```python
from build123d import *

# Parameters (mm, degrees)
ESBO_O1_W                = 30
ESBO_O1_H                = 22.5248
RESSALTO_EXTRUS_O1_DEPTH = 12.7
ESBO_O2_W                = 9.2624
ESBO_O2_H                = 20
CORTE_EXTRUS_O1_DEPTH    = 13.7
ESBO_O3_W                = 9.2624
ESBO_O3_H                = 20
CORTE_EXTRUS_O2_DEPTH    = 13.7
FURO1_D                  = 4.9784
FURO1_DEPTH              = 10
FURO1_CBORE_D            = 7.9375
FURO1_CBORE_DEPTH        = 4.1656
ESBO_O8_R                = 1.25
CORTE_EXTRUS_O3_DEPTH    = 10


with BuildPart() as part:
    # Esboço1 → Ressalto-extrusão1 (new body)
    with BuildSketch(Plane(origin=(0, 0, 0), x_dir=(0, -1, 0), z_dir=(-1, 0, 0))):
        with Locations((15, 11.2624)):
            Rectangle(ESBO_O1_W, ESBO_O1_H)
    extrude(amount=-RESSALTO_EXTRUS_O1_DEPTH)

    # Esboço2 → Corte-extrusão1 (cut, through all)
    with BuildSketch(Plane(origin=(12.7, 0, 0), x_dir=(0, 0, -1), z_dir=(1, 0, 0))):
        with Locations((-4.6312, -20)):
            Rectangle(ESBO_O2_W, ESBO_O2_H)
    extrude(amount=-CORTE_EXTRUS_O1_DEPTH, mode=Mode.SUBTRACT)

    # Esboço3 → Corte-extrusão2 (cut, through all)
    with BuildSketch(Plane(origin=(12.7, 0, 0), x_dir=(0, 0, -1), z_dir=(1, 0, 0))):
        with Locations((-17.8936, -20)):
            Rectangle(ESBO_O3_W, ESBO_O3_H)
    extrude(amount=-CORTE_EXTRUS_O2_DEPTH, mode=Mode.SUBTRACT)

    # Furo1
    with Locations(Plane(origin=(0, -10, 0), x_dir=(-1, 0, 0), z_dir=(0, -1, 0))):
        with Locations((-6.35, -4.6312), (-6.35, -17.8936)):
            CounterBoreHole(FURO1_D / 2, FURO1_CBORE_D / 2, FURO1_CBORE_DEPTH, depth=FURO1_DEPTH)

    # Esboço8 → Corte-extrusão3 (cut)
    with BuildSketch(Plane.XY.offset(13.2624)):
        with Locations((6.35, -15.143672471)):
            Circle(ESBO_O8_R)
        with Locations((6.35, -23.520600125)):
            Circle(ESBO_O8_R)
    extrude(amount=-CORTE_EXTRUS_O3_DEPTH, mode=Mode.SUBTRACT)


solid = part.part
```
Can you work these out from the model? Positions are in its coordinate system, mm. A direction names the side the tool comes from. Coordinates: 2 decimals unless noted, no trailing zeros. Loops run counter-clockwise (first coordinate to the right, second up) from the corner with the lowest first, then second, coordinate; pieces in that order, holes last. Notation, with made-up numbers: M -5.5,20.5 L 8.5,20.5 A29 cw 8.5,42.5 Z; hole C 59.25,4 d1. An arc over 180 degrees is marked long. Put each result on its own line as item: value. Start each with the question number.
(1) Will these pins go through, and if not, where does the flat tip stop? pin 1 Ø2.5 at (x, z) = (4.5, 18) entering from -Y; pin 2 Ø2 at (x, y) = (5, -15) entering from +Z; pin 3 Ø3 at (x, z) = (9, 19) entering from -Y.
(2) We'd pull the mould along Z, two halves only. Please class faces 4 (the face through (6, -5, 22.525)), 5 (the face through (12.7, -8, 11)), 6 (the face through (3.8, -5.834, 5.5)): +Z half, -Z half, draft (parallel to the pull), parting line (faces both ways), or undercut.
(3) Imagine slicing it at B-B on x = 6.35. Give the number of separate pieces and of enclosed holes in the cut face, and give its area (3 significant figures).
(4) Imagine slicing it at C-C on x = 2. List the corners of the cut face in (y, z) for me, and give its area (3 significant figures).
(5) Imagine slicing it at D-D on x = 4.25. List the corners of the cut face in (y, z) for me.
(6) Which directions (+Z, -Z, +X, -X, +Y, -Y) give clear straight access to the entire face, cutting with the end or side of a thin tool? Please do faces 1 (the face through (6, -10, 22)), 2 (the face through (6, -10, 9)), 3 (the face through (9.275, -7.946, 1.949)).
(7) I need wall thicknesses on probe 1 along Y at (x, z) = (6.35, 12.35); probe 2 along Z at (x, y) = (6.35, -2.6); probe 3 along Z at (x, y) = (6.35, -8.6). Which ranges of each line are inside material? Lowest first, please.
(8) Imagine slicing it at A-A on z = 2.5. List the corners of the cut face in (x, y) for me, and give its area (3 significant figures).
Worked answers:
1. pin 1: stops at y = -5.83
1. pin 2: stops at z = 13.26
1. pin 3: stops at y = -10
2. face 4: +Z half
2. face 5: draft
2. face 6: undercut
3. separate pieces: 5
3. enclosed holes: 0
3. area: 161 mm2
4. outline: M -30,9.26 L -10,9.26 L -10,0 L 0,0 L 0,22.52 L -10,22.52 L -10,13.26 L -30,13.26 Z
4. area: 305 mm2
5. outline: M -30,9.26 L -10,9.26 L -10,8 L -5.83,8 L -5.83,5.97 L 0,5.97 L 0,16.56 L -5.83,16.56 L -5.83,14.53 L -10,14.53 L -10,13.26 L -30,13.26 Z; M -10,0 L 0,0 L 0,3.29 L -5.83,3.29 L -5.83,1.26 L -10,1.26 Z; M -10,21.26 L -5.83,21.26 L -5.83,19.23 L 0,19.23 L 0,22.52 L -10,22.52 Z
6. face 1: +Z, +X, -X, -Y
6. face 2: -Z, +X, -X, -Y
6. face 3: -Y
7. probe 1: y = -30 to -24.77, -22.27 to -16.39, -13.89 to 0
7. probe 2: z = 0 to 2.14, 7.12 to 15.4, 20.38 to 22.52
7. probe 3: z = 0 to 0.66, 8.6 to 13.92, 21.86 to 22.52
8. outline: M 0,-10 L 3,-10 L 3,-5.83 L 5.06,-5.83 L 5.06,0 L 0,0 Z; M 7.64,-5.83 L 9.7,-5.83 L 9.7,-10 L 12.7,-10 L 12.7,0 L 7.64,0 Z
8. area: 84.1 mm2
